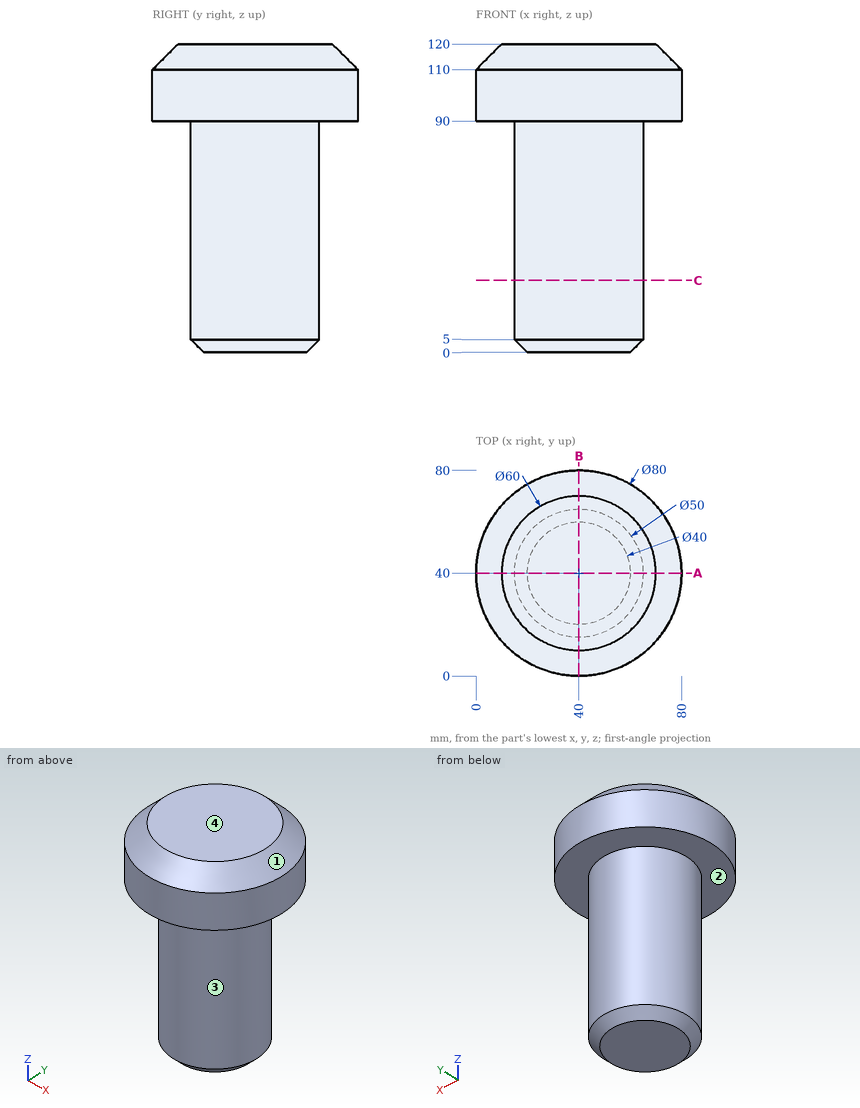
Answer from the drawing. Dimensions are ordinates in mm from the lowest x, y and z of the part. A direction names the side the tool comes from. Give positions to 0.01 mm unless a question says otherwise; leave off trailing zeros. Write each loop counter-clockwise with the first axis right and the second up, starting at its lowest first coordinate (ties: lowest second). Pieces come first, ordered by that corner, then holes. Notation, with made-up numbers: (-25, -38) -> (-8, -38) arc R26 cw to (-8, -17) -> close; hole circle Ø4 at (38, 49.5). An arc over 180 degrees is marked (long way). One line per question, with ' | ' between items. Start each with the question number.
1. For a pull along X with two mould halves and no side action, classify the marked faces 3 and 4 as pulls with the +X half, pulls with the -X half, needs draft (parallel to the pull), parting line crosses it, or undercut.
2. Given pin 1 Ø2 at (x, z) = (51, 65) entering from +Y; pin 2 Ø3 at (x, z) = (16.5, 15) entering from +Y; pin 3 Ø4 at (x, z) = (49.5, 75) entering from -Y, each flat-ended and moving along its own axis, determine where each tip first touches the part or whether it passes through.
3. Section A-A (y = 40) is taken. Determine the outline of the cut face in (x, z).
4. For the marked faces 1 and 2, determine the directions among +Z, -Z, +X, -X, +Y, -Y from which every point of the face is accessible in a straight line to the end or side of a thin tool.
5. Section C-C (z = 28) is taken. Determine the outline of the cut face in (x, y).
6. Find the intervals of material crossed by probe 1 along Y at (x, z) = (40, 48.5); probe 2 along Y at (x, z) = (37.5, 32); probe 3 along X at (y, z) = (53.5, 40), in increasing order.
Response values:
1) face 3: parting line crosses it | face 4: needs draft
2) pin 1: y = 62.91 | pin 2: y = 51.87 | pin 3: y = 16.15
3) outline: (0, 90) -> (15, 90) -> (15, 5) -> (20, 0) -> (60, 0) -> (65, 5) -> (65, 90) -> (80, 90) -> (80, 110) -> (70, 120) -> (10, 120) -> (0, 110) -> close
4) face 1: +Z | face 2: -Z
5) outline: circle Ø50 at (40, 40)
6) probe 1: 15 to 65 | probe 2: 15.13 to 64.87 | probe 3: 18.96 to 61.04
